from build123d import *

# Parameters (mm, degrees)
F0_W     = 60
F0_H     = 40
F1_DEPTH = 15
F2_T     = -5
F3_R     = 5


with BuildPart() as f1:
    # F0 (on Top) → F1 (new body)
    with BuildSketch(Plane.XY):
        Rectangle(F0_W, F0_H)
    extrude(amount=F1_DEPTH)

    # F2
    f2_openings = [f1.faces().sort_by_distance(p)[0] for p in [
        (0, 0, 15),
    ]]
    offset(amount=F2_T, openings=f2_openings)

    # F3
    f3_edges = [f1.edges().sort_by_distance(p)[0] for p in [
        (-30, 20, 7.5),
        (30, 20, 7.5),
        (-30, -20, 7.5),
        (30, -20, 7.5),
        (-25, -15, 10),
        (-25, 15, 10),
        (25, -15, 10),
        (25, 15, 10),
        (0, 20, 0),
        (0, -20, 0),
    ]]
    fillet(f3_edges, radius=F3_R)


solid = f1.part
Could you check a few things on this model? Use its own coordinates, in mm. A direction names the side the tool comes from. Give positions to 0.01 mm unless a question says otherwise; leave off trailing zeros. Loops run counter-clockwise (first coordinate to the right, second up) from the corner with the lowest first, then second, coordinate; pieces in that order, holes last. Notation, with made-up numbers: (72, 89.5) -> (113, 89.5) arc R22 ccw to (113, 118.5) -> close; hole circle Ø4 at (-20, 44.25). An arc over 180 degrees is marked (long way). Answer as CSV lines item,"result". Start each with the question number.
(1) If we section it at C-C on x = 12: Write out the boundary of the cut face in (y, z).
(2) I'm going to push flat-ended pins straight in: pin 1 Ø5 at (x, z) = (-14, 1.5) entering from +Y; pin 2 Ø15 at (x, y) = (-12, 1.5) entering from +Z. Where does each tip first touch, or does it pass through?
(3) I need wall thicknesses on probe 1 along Y at (x, z) = (-18.5, 10.25); probe 2 along X at (y, z) = (-0.5, 8.5); probe 3 along Z at (x, y) = (10, 3). Which ranges of each line are inside material? Lowest first, please.
(4) Which directions (+Z, -Z, +X, -X, +Y, -Y) give clear straight access to the entire face, cutting with the end or side of a thin tool? Please do faces 1 (the cylindrical face through (-24, 13, 10)), 2 (the flat face through (-30, 0, 7)).
(5) If we section it at D-D on z = 1: Write out the boundary of the cut face in (x, y).
(6) If we section it at A-A on z = 11: Write out the boundary of the cut face in (x, y).
(7) If we section it at B-B on y = 6: Write out the boundary of the cut face in (x, z).
(8) We'd pull the mould along X, two halves only. Please class faces 3 (the cylindrical face through (24, 13, 10)), 4 (the cylindrical face through (23, -14, 10)), 5 (the cylindrical face through (-29, -18, 8)), 6 (the flat face through (30, 0, 7)): released by +X, released by -X, zero draft, split by the parting line, or undercut.
Computed:
1,outline,"(-20, 5) arc R5 ccw to (-15, 0) -> (15, 0) arc R5 ccw to (20, 5) -> (20, 15) -> (15, 15) -> (15, 5) -> (-15, 5) -> (-15, 15) -> (-20, 15) -> close"
2,pin 1,"stops at y = 19.9"
2,pin 2,"stops at z = 5"
3,probe 1,"y = -20 to -15, 15 to 20"
3,probe 2,"x = -30 to -25, 25 to 30"
3,probe 3,"z = 0 to 5"
4,face 1,"+Z"
4,face 2,"+Z, -Z, -X, +Y, -Y"
5,outline,"(-30, -15) arc R5 ccw to (-29, -18) -> (29, -18) arc R5 ccw to (30, -15) -> (30, 15) arc R5 ccw to (29, 18) -> (-29, 18) arc R5 ccw to (-30, 15) -> close"
6,outline,"(-30, -15) arc R5 ccw to (-25, -20) -> (25, -20) arc R5 ccw to (30, -15) -> (30, 15) arc R5 ccw to (25, 20) -> (-25, 20) arc R5 ccw to (-30, 15) -> close; hole (-25, -10) arc R5 ccw to (-20, -15) -> (20, -15) arc R5 ccw to (25, -10) -> (25, 10) arc R5 ccw to (20, 15) -> (-20, 15) arc R5 ccw to (-25, 10) -> close"
7,outline,"(-30, 0) -> (30, 0) -> (30, 15) -> (25, 15) -> (25, 5) -> (-25, 5) -> (-25, 15) -> (-30, 15) -> close"
8,face 3,"undercut"
8,face 4,"undercut"
8,face 5,"released by -X"
8,face 6,"released by +X"
